Source: CAD feature listing. Evaluate the final solid. Frame: model axes, mm. Round coordinates to 2 decimals unless told otherwise and drop trailing zeros. Loops run counter-clockwise (first coordinate to the right, second up) from the corner with the lowest first, then second, coordinate; pieces in that order, holes last.
(1) Material intervals for probe 1 along Z at (x, y) = (11, 189); probe 2 along Z at (x, y) = (8.5, 236); probe 3 along Y at (x, z) = (10, -628.5), sorted ascending.
(2) First-contact query: pin 1 Ø1 at (x, y) = (9, 215) entering from -Z (3 decimals); pin 2 Ø4 at (x, y) = (11, 179) entering from -Z. Flat tips, straight axial feed; report the tip coordinate or a pass-through.
(3) Section A-A, the plane x = 7.75. Return the cut outline in (y, z), plus the area to 3 significant figures.
```python
from build123d import *

# Parameters (mm, degrees)
BOSS_EXTRUDE2_DEPTH = 12.7
CUT_EXTRUDE1_DEPTH  = 778.596755789
FILLET1_R           = 2.54


with BuildPart() as part:
    # Sketch1 → Boss-Extrude2 (new body)
    with BuildSketch(Plane(origin=(0, 0, 0), x_dir=(0, 0, -1), z_dir=(1, 0, 0))):
        Polygon((584.2, 304.8), (0, 304.8), (0, 0), (711.2, 0), align=None)
    extrude(amount=BOSS_EXTRUDE2_DEPTH)

    # Sketch3 → Cut-Extrude1 (cut, through all)
    with BuildSketch(Plane(origin=(11.214382214, 0, 4.081701322), x_dir=(0, 1, 0), z_dir=(0.9396926207859083, 0, 0.34202014332566943))):
        Polygon((304.8, -453.495658666), (152.4, -426.623426806), (152.4, -413.727508835), (304.8, -440.599740695), align=None)
    extrude(amount=-CUT_EXTRUDE1_DEPTH, mode=Mode.SUBTRACT)

    # Fillet1
    fillet1_edges = [part.edges().sort_by_distance(p)[0] for p in [
        (0, 304.8, -234.438225303),
        (0, 152.4, -647.7),
        (0, 152.4, 0),
        (12.7, 304.8, -232.127014316),
        (6.35, 304.8, -584.2),
        (6.35, 304.8, 0),
        (12.7, 152.4, 0),
        (12.7, 152.4, -647.7),
        (12.7, 304.8, -531.088788946),
        (0, 304.8, -533.399999933),
    ]]
    fillet(fillet1_edges, radius=FILLET1_R)


solid = part.part
```
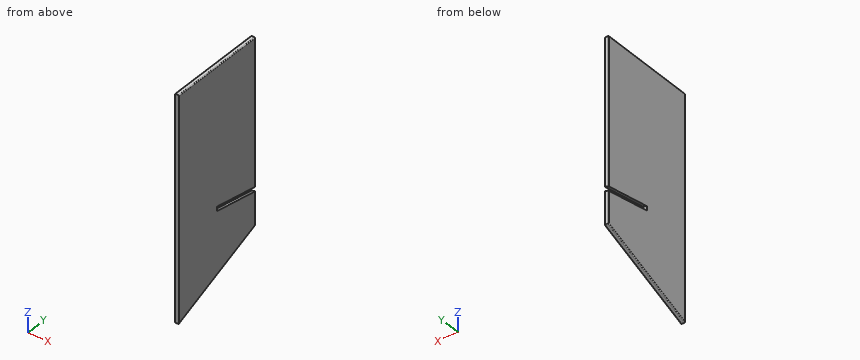
Output values:
1. probe 1: z = -632.3 to -456.87, -443.14 to -0.14
1. probe 2: z = -612.87 to -466.6, -452.87 to 0
1. probe 3: y = 0 to 198.48
2. pin 1: stops at z = -621.825
2. pin 2: stops at z = -637.4
3. outline: (0, -711.2) - (303.24, -584.85) arc R2.54 ccw to (304.8, -582.51) - (304.8, -479.78) - (152.4, -451.18) - (152.4, -437.46) - (304.8, -466.06) - (304.8, -2.54) arc R2.54 ccw to (302.26, 0) - (0, 0) - close
3. area: 195,000 mm2
